Study the drawing (mm; zero at the part's minimum x, y, z) and answer. Give positions to 0.01 mm unless a question says otherwise; leave off trailing zeros. Write each loop counter-clockwise with the first axis right and the second up, starting at its lowest first coordinate (ties: lowest second). Pieces come first, ordered by that corner, then holes.
1) Given pin 1 Ø0.5 at (x, z) = (8, 0.5) entering from -Y, flat-ended and moving along its own axis, determine where the tip first touches the part or whether it passes through.
2) Find section A-A (x = 4.25). Determine the outline of the cut face in (y, z).
3) Determine the mould class of the marked faces 1, 2 and 3 for opening direction Y: pulls with the +Y half, pulls with the -Y half, needs draft (parallel to the pull), parting line crosses it, or undercut.
4) Straight lines are drawn through the part: probe 1 along X at (y, z) = (0.5, 1.7) (1 decimal); probe 2 along Z at (x, y) = (6, 1.35); probe 3 along X at (y, z) = (1.45, 1.5). For each, find the intervals that lie inside material, in ascending order.
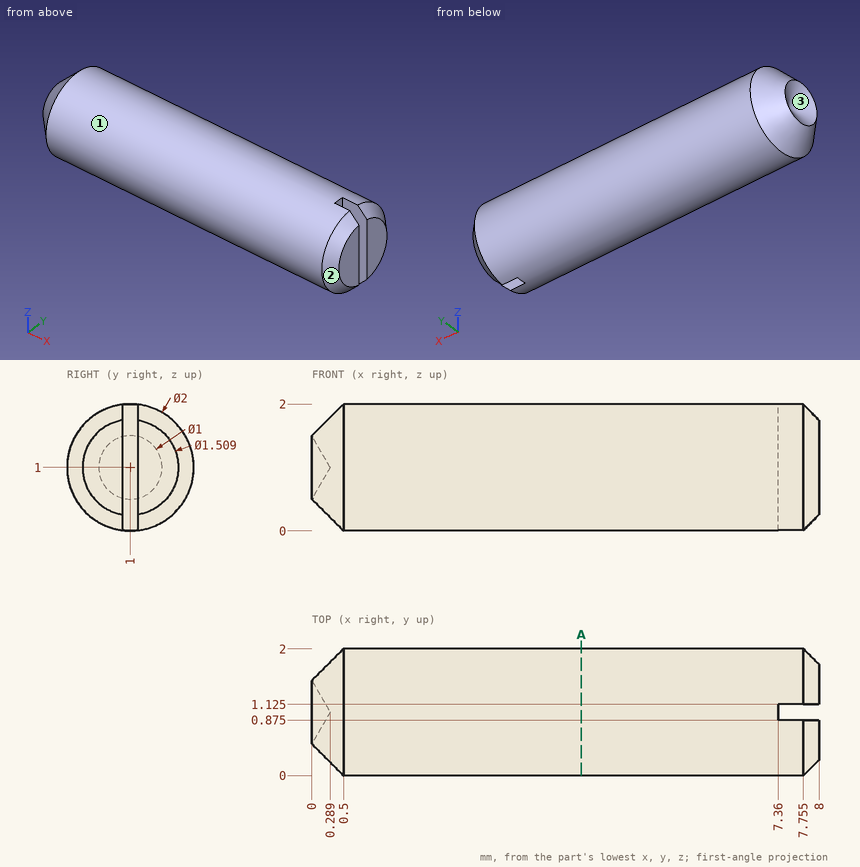
Results:
1. pin 1: stops at y = 0.1
2. outline: circle Ø2 at (1, 1)
3. face 1: parting line crosses it
3. face 2: pulls with the -Y half
3. face 3: undercut
4. probe 1: x = 0.4 to 7.9
4. probe 2: z = 0.06 to 1.94
4. probe 3: x = 0.17 to 8
